```python
from build123d import *

# Parameters (mm, degrees)
SKETCH1_W           = 138.5
SKETCH1_H           = 63.5
BOSS_EXTRUDE1_DEPTH = 6.35
SKETCH2_R           = 3.175
CUT_EXTRUDE1_DEPTH  = 6.35
FILLET1_R           = 10
CUT_EXTRUDE4_DEPTH  = 6.35


with BuildPart() as part:
    # Sketch1 → Boss-Extrude1 (new body)
    with BuildSketch(Plane(origin=(0, 0, 0), x_dir=(1, 0, 0), z_dir=(0, 1, 0))):
        Rectangle(SKETCH1_W, SKETCH1_H)
    extrude(amount=BOSS_EXTRUDE1_DEPTH)

    # Sketch2 → Cut-Extrude1 (cut)
    with BuildSketch(Plane(origin=(0, 6.35, 0), x_dir=(1, 0, 0), z_dir=(0, 1, 0))):
        with Locations((-54.9625, 17.4625)):
            Circle(SKETCH2_R)
        with Locations((-20.0375, 17.4625)):
            Circle(SKETCH2_R)
        with Locations((20.0375, 17.4625)):
            Circle(SKETCH2_R)
        with Locations((54.9625, 17.4625)):
            Circle(SKETCH2_R)
        with Locations((54.9625, -17.4625)):
            Circle(SKETCH2_R)
        with Locations((20.0375, -17.4625)):
            Circle(SKETCH2_R)
        with Locations((-20.0375, -17.4625)):
            Circle(SKETCH2_R)
        with Locations((-54.9625, -17.4625)):
            Circle(SKETCH2_R)
    extrude(amount=-CUT_EXTRUDE1_DEPTH, mode=Mode.SUBTRACT)

    # Fillet1
    fillet1_edges = [part.edges().sort_by_distance(p)[0] for p in [
        (69.25, 3.175, 31.75),
        (-69.25, 3.175, 31.75),
        (-69.25, 3.175, -31.75),
        (69.25, 3.175, -31.75),
    ]]
    fillet(fillet1_edges, radius=FILLET1_R)

    # Sketch3 → Cut-Extrude4 (cut)
    with BuildSketch(Plane(origin=(0, 6.35, 0), x_dir=(1, 0, 0), z_dir=(0, 1, 0))):
        with BuildLine():
            Line((-12.7, 31.75), (12.7, 31.75))
            ThreePointArc((12.7, 31.75), (0, 19.05), (-12.7, 31.75))
        make_face()
    extrude(amount=-CUT_EXTRUDE4_DEPTH, mode=Mode.SUBTRACT)


solid = part.part
```
The listing builds one solid part. Answer for the finished solid, in the listing's coordinates (mm). Coordinates: 2 decimals unless noted, no trailing zeros. Loops run counter-clockwise (first coordinate to the right, second up) from the corner with the lowest first, then second, coordinate; pieces in that order, holes last. Notation, with made-up numbers: (79, -33.75) - (118, -33.75) arc R15 ccw to (118, -7.75) - close; hole circle Ø9 at (83, 59). An arc over 180 degrees is marked (long way). Write item = value, one per line.
1) Each of these flat-tipped pins is pushed along its axis until it touches: P1, Ø5, axis at x = 20.04, z = 17.46, coming from the +Y side; P2, Ø12, axis at x = -7.5, z = 22, coming from the -Y side. Where does it stop, or does it pass through?
Responses:
P1 = through
P2 = 0
2) Section A-A (z = -23.5) is taken. Determine the outline of the cut face in (x, y), plus the area to 3 significant figures.
Responses:
outline = (-69.1, 0) - (-9.66, 0) - (-9.66, 6.35) - (-69.1, 6.35) - close; (9.66, 0) - (69.1, 0) - (69.1, 6.35) - (9.66, 6.35) - close
area = 755 mm^2
3) Section B-B (x = -20) is taken. Determine the outline of the cut face in (y, z), plus the area to 3 significant figures.
Responses:
outline = (0, -31.75) - (6.35, -31.75) - (6.35, -20.64) - (0, -20.64) - close; (0, -14.29) - (6.35, -14.29) - (6.35, 14.29) - (0, 14.29) - close; (0, 20.64) - (6.35, 20.64) - (6.35, 31.75) - (0, 31.75) - close
area = 323 mm^2
4) Section C-C (y = 2.75) is taken. Count the separate pieces of the cut face and the enclosed holes in it, plus the area to 3 significant figures.
Responses:
separate_pieces = 1
enclosed_holes = 8
area = 8,200 mm^2
5) Find the intervals of material crossed by line 1 along X through (y, z) = (4, -19); line 2 along Z through (x, y) = (-52.5, 2.5); line 3 along X through (y, z) = (3.5, 16.5), in increasing order.
Responses:
line_1 = -69.25 to -57.74, -52.18 to -22.82, -17.26 to 17.26, 22.82 to 52.18, 57.74 to 69.25
line_2 = -31.75 to -19.47, -15.46 to 15.46, 19.47 to 31.75
line_3 = -69.25 to -57.99, -51.94 to -23.06, -17.01 to 17.01, 23.06 to 51.94, 57.99 to 69.25
6) Determine the mould class of faces 1 (the face through (-36, 3, -31.75)), 2 (the face through (21.744, 3.219, -20.14)), 3 (the face through (-66.4, 3.22, -28.74)) for opening direction X: pulls with the +X half, pulls with the -X half, needs draft (parallel to the pull), parting line crosses it, or undercut.
Responses:
face_1 = needs draft
face_2 = undercut
face_3 = pulls with the -X half
7) Section D-D (x = 0) is taken. Determine the outline of the cut face in (y, z).
Responses:
outline = (0, -19.05) - (6.35, -19.05) - (6.35, 31.75) - (0, 31.75) - close
